from build123d import *

# Parameters (mm, degrees)
FILLET1_R                      = 1
FILLET2_R                      = 2
CUT_EXTRUDE1_REACH             = 23
F_4_1_4_1_DIAMETER_HOLE1_D     = 4.1
F_4_1_4_1_DIAMETER_HOLE1_DEPTH = 0.8


with BuildPart() as part:
    # Sketch1 → Revolve1 (revolve)
    with BuildSketch(Plane.XY):
        with BuildLine():
            Line((14, 1.7), (14, -8.3))
            Line((14, -8.3), (11.878679656, -10.421320344))
            Line((11.878679656, -10.421320344), (10.378679656, -13.019396555))
            Line((10.378679656, -13.019396555), (7.223021359, -13.019396555))
            ThreePointArc((7.223021359, -13.019396555), (4.533460369, -16.974758328), (0, -18.5))
            Line((0, -18.5), (0, 0))
            ThreePointArc((0, 0), (5.941029682, -1.742345528), (10, -6.417424305))
            Line((10, -6.417424305), (12, -6.417424305))
            Line((12, -6.417424305), (12, 2.5))
            Line((12, 2.5), (25, 2.5))
            Line((25, 2.5), (25, 1.7))
            Line((25, 1.7), (14, 1.7))
        make_face()
    revolve(axis=Axis((0, 43.298682787, 0), (0, -1, 0)))

    # Fillet1
    fillet1_edges = [part.edges().sort_by_distance(p)[0] for p in [
        (-7.223021359, -13.019396555, 0),
        (-10.378679656, -13.019396555, 0),
        (-11.878679656, -10.421320344, 0),
        (-14, -8.3, 0),
        (-14, 1.7, 0),
    ]]
    fillet(fillet1_edges, radius=FILLET1_R)

    # Fillet2
    fillet2_edges = [part.edges().sort_by_distance(p)[0] for p in [
        (-12, 2.5, 0),
    ]]
    fillet(fillet2_edges, radius=FILLET2_R)

    # Sketch2 → Cut-Extrude1 (cut, up to next)
    with BuildSketch(Plane(origin=(0, 2.5, 0), x_dir=(1, 0, 0), z_dir=(0, 1, 0)), mode=Mode.PRIVATE) as cut_extrude1_sk1:
        with BuildLine():
            ThreePointArc((-25, 0), (-24.437059837, 2.304886114), (-22.875, 4.090767043))
            Line((-22.875, 4.090767043), (-9.4875, 13.499531242))
            ThreePointArc((-9.4875, 13.499531242), (0, 16.5), (9.4875, 13.499531242))
            Line((9.4875, 13.499531242), (22.875, 4.090767043))
            ThreePointArc((22.875, 4.090767043), (24.437059837, 2.304886114), (25, 0))
            ThreePointArc((25, 0), (0, 25), (-25, 0))
        make_face()
    cut_extrude1_tool1 = extrude(cut_extrude1_sk1.sketch, amount=-CUT_EXTRUDE1_REACH, mode=Mode.PRIVATE) & part.part
    add(cut_extrude1_tool1.solids().sort_by_distance((-24.486668, 2.5, -2.330656))[0], mode=Mode.SUBTRACT)
    # Sketch2 → Cut-Extrude1 (cut, up to next)
    with BuildSketch(Plane(origin=(0, 2.5, 0), x_dir=(1, 0, 0), z_dir=(0, 1, 0)), mode=Mode.PRIVATE) as cut_extrude1_sk2:
        with BuildLine():
            ThreePointArc((-22.875, -4.090767043), (-24.437059837, -2.304886114), (-25, 0))
            ThreePointArc((-25, 0), (0, -25), (25, 0))
            ThreePointArc((25, 0), (24.437059837, -2.304886114), (22.875, -4.090767043))
            Line((22.875, -4.090767043), (9.4875, -13.499531242))
            ThreePointArc((9.4875, -13.499531242), (0, -16.5), (-9.4875, -13.499531242))
            Line((-9.4875, -13.499531242), (-22.875, -4.090767043))
        make_face()
    cut_extrude1_tool2 = extrude(cut_extrude1_sk2.sketch, amount=-CUT_EXTRUDE1_REACH, mode=Mode.PRIVATE) & part.part
    add(cut_extrude1_tool2.solids().sort_by_distance((-16.502685, 2.5, 9.252511))[0], mode=Mode.SUBTRACT)

    # Ø4.1 (4.1) Diameter Hole1
    with Locations(Plane(origin=(0, 2.5, 0), x_dir=(1, 0, 0), z_dir=(0, 1, 0))):
        with Locations((20, 0), (-20, 0)):
            Hole(F_4_1_4_1_DIAMETER_HOLE1_D / 2, depth=F_4_1_4_1_DIAMETER_HOLE1_DEPTH)


solid = part.part
Source: CAD feature listing. Evaluate the final solid. Frame: model axes, mm. A direction names the side the tool comes from. Give positions to 0.01 mm unless a question says otherwise; leave off trailing zeros. Write each loop counter-clockwise with the first axis right and the second up, starting at its lowest first coordinate (ties: lowest second). Pieces come first, ordered by that corner, then holes. Notation, with made-up numbers: (-12.75, 77.25) - (39.25, 77.25) arc R27 ccw to (39.25, 104.25) - close; hole circle Ø2 at (3, 22). An arc over 180 degrees is marked (long way). Write item = value, one per line. Start each with the question number.
Q1. Cut plane A-A, the plane x = -20. Return loops of the section in (y, z).
Q2. Cut plane C-C, the plane x = 19. Return loops of the section in (y, z).
Q3. Cut plane D-D, the plane y = -12. Return loops of the section in (x, z).
Q4. Reachability of faces 1 (the flat face through (5, -6.417, 9)), 2 (the cylindrical face through (-17.95, 2.09, -0.09)), 3 (the cylindrical face through (12.932, -3.653, -5.362)) from +Z, -Z, +X, -X, +Y, -Y: full face, straight path, thin tool, end or side. Return the list, or none.
Q5. Draft query along Z for faces 4 (the flat face through (-1.5, -13.019, 8)), 5 (the cylindrical face through (22.05, 2.09, -0.09)), 6 (the flat face through (-16.275, 2.106, -8.729)). Return one class per face: +Z half, -Z half, draft (parallel to the pull), parting line (faces both ways), or undercut.
Q6. Cut plane B-B, the plane y = -4.5. Return loops of the section in (x, z), then the cut area to 3 significant figures.
Q7. Pin query (flat end, axial travel): pin 1 Ø2 at (x, y) = (-3, -1.5) entering from +Z; pin 2 Ø8 at (x, z) = (-7.5, 9) entering from -Y; pin 3 Ø10 at (x, z) = (7.5, 1.5) entering from -Y. Return the tip coordinate at first contact, or that it passes through.
Q8. Material intervals for probe 1 along Z at (x, y) = (-8, -5.5); probe 2 along Z at (x, y) = (-2.5, -5.75); probe 3 along Z at (x, y) = (3, 1.25), sorted ascending.
Computed values:
q1.outline = (1.7, -6.11) - (2.5, -6.11) - (2.5, -2.05) - (1.7, -2.05) - close; (1.7, 2.05) - (2.5, 2.05) - (2.5, 6.11) - (1.7, 6.11) - close
q2.outline = (1.7, -6.81) - (2.5, -6.81) - (2.5, -1.79) - (1.7, -1.79) - close; (1.7, 1.79) - (2.5, 1.79) - (2.5, 6.81) - (1.7, 6.81) - close
q3.outline = circle Ø21.93 at (0, 0)
q4.face_1 = +Y
q4.face_2 = +Y, -Y
q4.face_3 = -Y
q5.face_4 = draft
q5.face_5 = undercut
q5.face_6 = -Z half
q6.outline = circle Ø28 at (0, 0); circle Ø17.75 at (0, 0); hole circle Ø24 at (0, 0)
q6.area = 411 mm²
q7.pin_1 = 13.86
q7.pin_2 = -13.05
q7.pin_3 = -18.02
q8.probe_1 = -11.49 to -8.94, -5.17 to 5.17, 8.94 to 11.49
q8.probe_2 = -13.77 to -11.74, -9.34 to 9.34, 11.74 to 13.77
q8.probe_3 = -13.84 to -11.77, 11.77 to 13.84
